For this review, take the finished solid that the model builds, in its own axes (mm). A direction names the side the tool comes from. Coordinates: 2 decimals unless noted, no trailing zeros. Loops run counter-clockwise (first coordinate to the right, second up) from the corner with the lowest first, then second, coordinate; pieces in that order, holes last. Notation, with made-up numbers: (69.5, 41.25) - (121.5, 41.25) arc R34 cw to (121.5, 79.25) - close; hole circle Ø11 at (33, 14). An arc over 180 degrees is marked (long way). Answer as a JSON object with one key per item and string values. Group by question number.
Item 1: To check wall thickness, follow line 1 (X direction, y = -2.75, z = 21); line 2 (Y direction, x = 15.5, z = 0); line 3 (Y direction, x = 8.5, z = 3). State the ranges of each line that lie inside material, in increasing order.
Item 2: We need section B-B (y = -5.5). Give the boundary of the cut face in (x, z), then the cut area to 3 significant figures.
Item 3: We need section D-D (z = 17). Give the boundary of the cut face in (x, y), then the cut area to 3 significant figures.
Item 4: Mouldability with a two-part tool opening along X and no side actions: class faces 1 (the flat face through (-25, -3, 0)), 2 (the flat face through (20, 0, 0)), 3 (the cylindrical face through (-4.42, 5.97, -0.46)) as released by +X, released by -X, zero draft, split by the parting line, or undercut.
Item 5: Clearance check with flat-ended pins moving along their axes: pin 1 (3 mm diameter, centred on y = -6, z = 17, fed in from -X); pin 2 (1 mm diameter, centred on x = -4, y = -3, fed in from -Z); pin 3 (3 mm diameter, centred on x = 21, z = -1, fed in from -Y); pin 4 (4 mm diameter, centred on x = 16, y = 4.5, fed in from -Z). State where each tip first meets the part, or that it passes through.
Item 6: We need section C-C (z = 0). Give the boundary of the cut face in (x, y), then the cut area to 3 significant figures.
Item 7: We need section A-A (x = 0). Give the boundary of the cut face in (y, z), then the cut area to 3 significant figures.
Item 8: Tool access review of faces 4 (the flat face through (15, -5, 0)), 5 (the flat face through (-6, 4, 2)), 6 (the flat face through (-20, 1, 5)): name each direction out of +Z, -Z, +X, -X, +Y, -Y from which nothing blocks a thin tool from reaching the whole face with its end or side.
from build123d import *

# Parameters (mm, degrees)
EXTRUDE_1_DEPTH     = 4
SKETCH_1_W          = 10
SKETCH_1_H          = 10
EXTRUDE_2_DEPTH     = 10
SKETCH_3_W          = 6
SKETCH_3_H          = 12.745836759
SKETCH_3_H_2        = 13.387334875
CUT_EXTRUDE_1_DEPTH = 28
CUT_EXTRUDE_2_DEPTH = 51
SKETCH_5_R          = 6
EXTRUDE_3_DEPTH     = 4


with BuildPart() as part:
    # 草图2 → 凸台-拉伸1 (new body)
    with BuildSketch(Plane(origin=(0, 0, 0), x_dir=(1, 0, 0), z_dir=(0, 1, 0))):
        Polygon((-5, -22), (5, -22), (5, -12), (15, -5), (25, -5), (25, 5), (-25, 5), (-25, -5), (-15, -5), (-5, -12), align=None)
    extrude(amount=EXTRUDE_1_DEPTH)

    # 草图1 → 凸台-拉伸2 (add)
    with BuildSketch(Plane(origin=(0, 0, 0), x_dir=(1, 0, 0), z_dir=(0, 1, 0))):
        with Locations((-20, 0)):
            Rectangle(SKETCH_1_W, SKETCH_1_H)
        with Locations((20, 0)):
            Rectangle(SKETCH_1_W, SKETCH_1_H)
        with Locations((0, -17)):
            Rectangle(SKETCH_1_W, SKETCH_1_H)
    extrude(amount=-EXTRUDE_2_DEPTH)

    # 草图3 → 切除-拉伸1 (cut, through all)
    with BuildSketch(Plane(origin=(0, 0, -5), x_dir=(-1, 0, 0), z_dir=(0, 0, -1))):
        with Locations((-20, -6.37291838)):
            Rectangle(SKETCH_3_W, SKETCH_3_H)
        with Locations((0, -6.37291838)):
            Rectangle(SKETCH_3_W, SKETCH_3_H)
        with Locations((20, -6.693667438)):
            Rectangle(SKETCH_3_W, SKETCH_3_H_2)
    extrude(amount=-CUT_EXTRUDE_1_DEPTH, mode=Mode.SUBTRACT)

    # 草图4 → 切除-拉伸2 (cut, through all)
    with BuildSketch(Plane(origin=(25, 0, 0), x_dir=(0, 0, -1), z_dir=(1, 0, 0))):
        with BuildLine():
            Line((-22, -5), (-22, -12.80603889))
            Line((-22, -12.80603889), (-12, -12.80603889))
            Line((-12, -12.80603889), (-12, -5))
            ThreePointArc((-12, -5), (-17, -10), (-22, -5))
        make_face()
        with BuildLine():
            Line((-5, -5), (-5, -13.738678459))
            Line((-5, -13.738678459), (5, -13.738678459))
            Line((5, -13.738678459), (5, -5))
            ThreePointArc((5, -5), (0, -10), (-5, -5))
        make_face()
    extrude(amount=-CUT_EXTRUDE_2_DEPTH, mode=Mode.SUBTRACT)

    # 草图5 → 凸台-拉伸3 (add)
    with BuildSketch(Plane(origin=(0, 4, 0), x_dir=(1, 0, 0), z_dir=(0, 1, 0))):
        with Locations((0, -3.6)):
            Circle(SKETCH_5_R)
    extrude(amount=EXTRUDE_3_DEPTH)


solid = part.part
Check sheet entries:
{
 "1": {"line 1": "x = -5 to -3, 3 to 5", "line 2": "y = -10 to 4", "line 3": "y = 0 to 4"},
 "2": {"outline": "(-25, -4.97) - (-23, -4.97) - (-23, 4.97) - (-25, 4.97) - close; (-17, -4.97) - (-15, -4.97) - (-15, 4.97) - (-17, 4.97) - close; (-5, 12.03) - (-3, 12.03) - (-3, 21.97) - (-5, 21.97) - close; (3, 12.03) - (5, 12.03) - (5, 21.97) - (3, 21.97) - close; (15, -4.97) - (17, -4.97) - (17, 4.97) - (15, 4.97) - close; (23, -4.97) - (25, -4.97) - (25, 4.97) - (23, 4.97) - close", "area": "119 mm2"},
 "3": {"outline": "(-5, -10) - (-3, -10) - (-3, 0) - (3, 0) - (3, -10) - (5, -10) - (5, 4) - (-5, 4) - close", "area": "80.0 mm2"},
 "4": {"face 1": "released by -X", "face 2": "undercut", "face 3": "split by the parting line"},
 "5": {"pin 1": "stops at x = -5", "pin 2": "stops at z = 12", "pin 3": "stops at y = 0", "pin 4": "stops at z = -5"},
 "6": {"outline": "(-25, -10) - (-23, -10) - (-23, 0) - (-17, 0) - (-17, -10) - (-15, -10) - (-15, 0) - (15, 0) - (15, -10) - (17, -10) - (17, 0) - (23, 0) - (23, -10) - (25, -10) - (25, 4) - (4.8, 4) - (4.8, 8) - (-4.8, 8) - (-4.8, 4) - (-25, 4) - close", "area": "318 mm2"},
 "7": {"outline": "(0, -5) - (4, -5) - (4, -2.4) - (8, -2.4) - (8, 9.6) - (4, 9.6) - (4, 22) - (0, 22) - close", "area": "156 mm2"},
 "8": {"face 4": "+Z, -Z, -Y", "face 5": "+Y", "face 6": "+Z, -X, +Y, -Y"}
}
